from build123d import *

# Parameters (mm, degrees)
F0_R     = 25.4
F1_DEPTH = 254
F2_SIZE  = 5.08
F3_T     = -2.54


with BuildPart() as f1:
    # F0 (on Front) → F1 (new body)
    with BuildSketch(Plane.XZ):
        Circle(F0_R)
    extrude(amount=F1_DEPTH)

    # F2
    f2_edges = [f1.edges().sort_by_distance(p)[0] for p in [
        (-25.4, -254, 0),
    ]]
    chamfer(f2_edges, length=F2_SIZE)

    # F3
    f3_openings = [f1.faces().sort_by_distance(p)[0] for p in [
        (0, -254, 0),
    ]]
    offset(amount=F3_T, openings=f3_openings)


solid = f1.part
Here's how the part is built. I have some questions about the finished solid (model axes, mm). A direction names the side the tool comes from. Coordinates: 2 decimals unless noted, no trailing zeros. Order: outer loops, then holes, each group sorted by start corner. A loop starts at its lowest first (then second) coordinate and runs counter-clockwise, first axis right, second up. Notation, with made-up numbers: M -5.5,-14 L 9.5,-14 A30 ccw 9.5,18 Z; hole C 27,85.25 d2. An arc over 180 degrees is marked long. Answer as CSV lines item,"result".
Item 1: For pin 1 (3 mm diameter, centred on x = 0.5, y = -160.5, fed in from +Z); pin 2 (3 mm diameter, centred on y = -114, z = -6, fed in from +X); pin 3 (4 mm diameter, centred on y = -101.5, z = 18.5, fed in from +X), each with a flat end and sliding along its axis, tell me the tip position at first contact or that it passes through.
Results found:
pin 1,"z = 25.4"
pin 2,"x = 25"
pin 3,"x = 19.31"
Item 2: Imagine slicing it at A-A on y = -60.5. Write out the boundary of the cut face in (x, z), plus the area to 3 significant figures.
Results found:
outline,"C 0,0 d50.8; hole C 0,0 d45.72"
area,"385 mm2"
Item 3: If I drill on line 1 (Z direction, x = 0, y = -91); line 2 (X direction, y = -105.5, z = -21); line 3 (Y direction, x = 15, z = -6), over which ranges is the centre line in solid material (lowest first)?
Results found:
line 1,"-25.4 to -22.86, 22.86 to 25.4"
line 2,"-14.29 to -9.03, 9.03 to 14.29"
line 3,"-2.54 to 0"
Item 4: Imagine slicing it at B-B on z = 0. Write out the boundary of the cut face in (x, y), plus the area to 3 significant figures.
Results found:
outline,"M -25.4,-248.92 L -20.32,-254 L -16.73,-254 L -22.86,-247.87 L -22.86,-2.54 L 22.86,-2.54 L 22.86,-247.87 L 16.73,-254 L 20.32,-254 L 25.4,-248.92 L 25.4,0 L -25.4,0 Z"
area,"1,420 mm2"
Item 5: Imagine slicing it at C-C on x = 0. Write out the boundary of the cut face in (y, z), plus the area to 3 significant figures.
Results found:
outline,"M -254,-20.32 L -248.92,-25.4 L 0,-25.4 L 0,25.4 L -248.92,25.4 L -254,20.32 L -254,16.73 L -247.87,22.86 L -2.54,22.86 L -2.54,-22.86 L -247.87,-22.86 L -254,-16.73 Z"
area,"1,420 mm2"
Item 6: We'd pull the mould along X, two halves only. Please class faces 1 (the face through (0, -2.54, 0)), 2 (the face through (0, 0, 0)), 3 (the face through (-5.506, -122.718, -24.796)): +X half, -X half, draft (parallel to the pull), parting line (faces both ways), or undercut.
Results found:
face 1,"undercut"
face 2,"draft"
face 3,"parting line"
Item 7: On a 3-axis mill with a long thin cutter (end or side, diameter ignored), from which of +Z, -Z, +X, -X, +Y, -Y can I reach the whole of each face in a straight line? I mean faces 4 (the face through (-13.511, -253.702, -10.36)), 5 (the face through (-16.321, -253.753, -12.514)). Say none if no direction works.
Results found:
face 4,"none"
face 5,"-Y"
